Source: three-view drawing plus pictorial views. Frame: mm from the lowest corner of the part. A direction names the side the tool comes from. Give positions to 0.01 mm unless a question says otherwise; leave off trailing zeros. Write each loop counter-clockwise with the first axis right and the second up, starting at its lowest first coordinate (ties: lowest second). Pieces come first, ordered by that corner, then holes.
Q1. Pin query (flat end, axial travel): pin 1 (3 mm diameter, centred on x = 5, z = 7, fed in from +Y); pin 2 (2 mm diameter, centred on x = 8, z = 1.5, fed in from -Y); pin 3 (2 mm diameter, centred on x = 7, y = 2, fed in from -Z). Return the tip coordinate at first contact, or that it passes through.
Q2. Cut plane B-B on z = 8.25. Return the cut outline in (x, y).
Q3. Line query: L1, parallel to Y at x = 7.5, z = 11; L2, parallel to X at y = 27, z = 10.5; L3, parallel to Y at x = 3.75, z = 2.25. Output: solid intervals per line, ascending.
Q4. Draft query along Y for the marked faces 1, 2 and 3. Return one class per face: pulls with the +Y half, pulls with the -Y half, needs draft (parallel to the pull), parting line crosses it, or undercut.
Q5. Cut plane D-D on y = 6.5. Return the cut outline in (x, z), plus the area to 3 significant figures.
Q6. Cut plane A-A on x = 5. Return the cut outline in (y, z).
Q7. Reachability of the marked faces 4, 5 and 6 from +Z, -Z, +X, -X, +Y, -Y: full face, straight path, thin tool, end or side. Return the list, or none.
Q8. Cut plane C-C on y = 3. Return the cut outline in (x, z), plus the area to 3 significant figures.
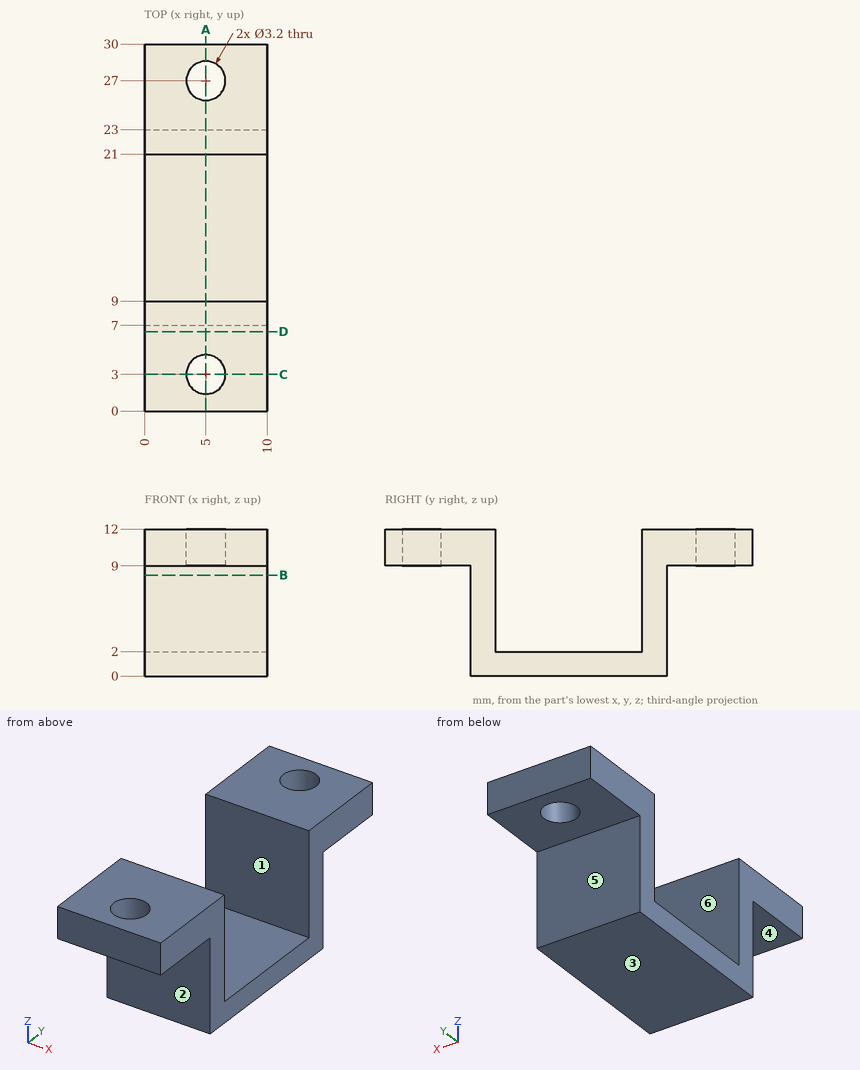
Data:
1. pin 1: stops at y = 23
1. pin 2: stops at y = 7
1. pin 3: stops at z = 9
2. outline: (0, 7) - (10, 7) - (10, 9) - (0, 9) - close; (0, 21) - (10, 21) - (10, 23) - (0, 23) - close
3. L1: y = 0 to 9, 21 to 30
3. L2: x = 0 to 3.4, 6.6 to 10
3. L3: y = 7 to 9, 21 to 23
4. face 1: undercut
4. face 2: pulls with the -Y half
4. face 3: needs draft
5. outline: (0, 9) - (10, 9) - (10, 12) - (0, 12) - close
5. area: 30.0 mm2
6. outline: (0, 9) - (1.4, 9) - (1.4, 12) - (0, 12) - close; (4.6, 9) - (7, 9) - (7, 0) - (23, 0) - (23, 9) - (25.4, 9) - (25.4, 12) - (21, 12) - (21, 2) - (9, 2) - (9, 12) - (4.6, 12) - close; (28.6, 9) - (30, 9) - (30, 12) - (28.6, 12) - close
7. face 4: -Z, +X, -X, -Y
7. face 5: -Z, +X, -X, +Y
7. face 6: +Z, +X, -X
8. outline: (0, 9) - (3.4, 9) - (3.4, 12) - (0, 12) - close; (6.6, 9) - (10, 9) - (10, 12) - (6.6, 12) - close
8. area: 20.4 mm2
